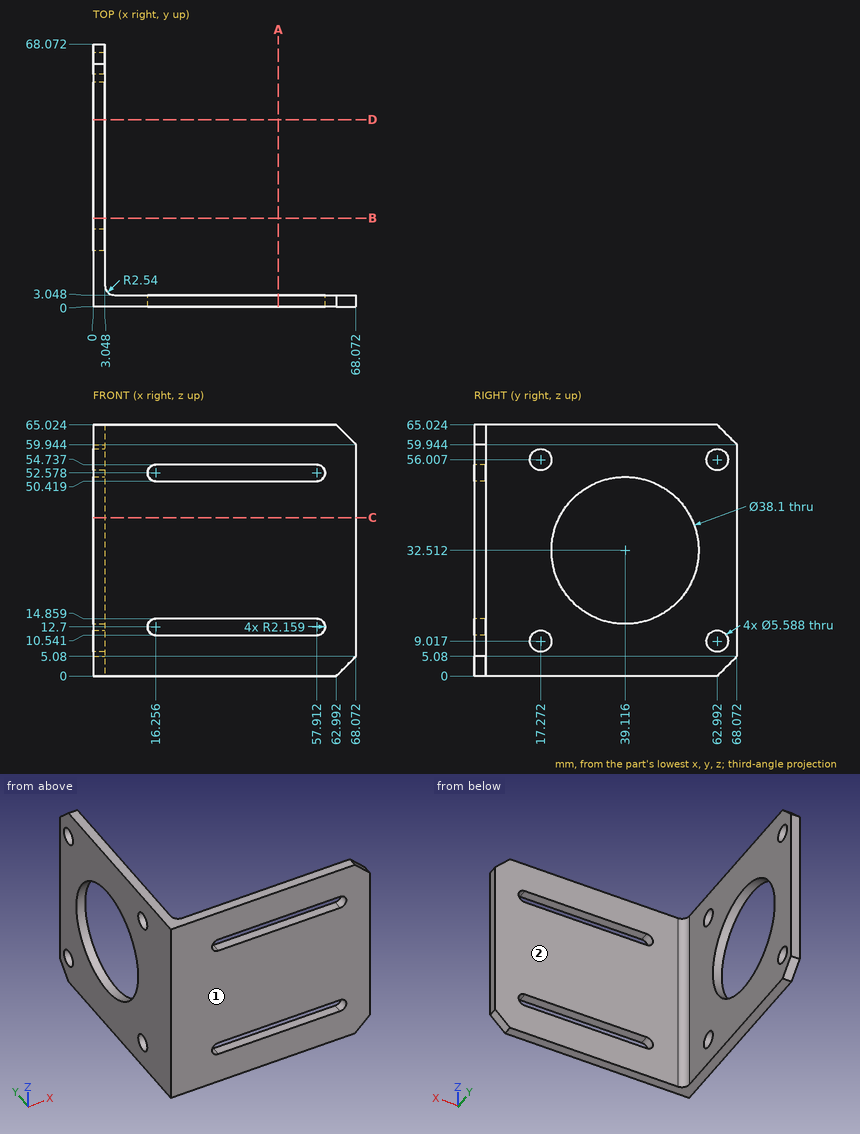
The figure shows three views and two pictorial views of one solid part (mm, origin at its lowest corner). Answer the questions. A direction names the side the tool comes from. Give positions to 0.01 mm unless a question says otherwise; leave off trailing zeros. Write each loop counter-clockwise with the first axis right and the second up, starting at its lowest first coordinate (ties: lowest second). Pieces come first, ordered by that corner, then holes. Notation, with made-up numbers: (-38.5, -12.5) - (-14.5, -12.5) arc R17 cw to (-14.5, -2.5) - close; hole circle Ø6 at (-38.75, -36). An arc over 180 degrees is marked (long way). Use CSV: the item, a comma, the result in double quotes. Start each with the question number.
Item 1: The part is cut by section A-A, the plane x = 48. Give the vertices of the cut face in (y, z).
Item 2: For the marked faces 1 and 2, determine the directions among +Z, -Z, +X, -X, +Y, -Y from which every point of the face is accessible in a straight line to the end or side of a thin tool.
Item 3: Consider line 1 (X direction, y = 61, z = 36); line 2 (X direction, y = 3.5, z = 44). Determine where each line is inside the solid, lowest interval first.
Item 4: Flat-ended cylindrical pins translate along their axes: P1, Ø1, axis at x = 25, z = 31.5, coming from the +Y side; P2, Ø9, axis at y = 62.992, z = 9.017, coming from the +X side. Find the tip coordinate at first contact, or state that the pin passes through.
Item 5: The part is cut by section B-B, the plane y = 23. Give the vertices of the cut face in (x, z), and give its area (3 significant figures).
Item 6: The part is cut by section D-D, the plane y = 48.5. Give the vertices of the cut face in (x, z), and give its area (3 significant figures).
Item 7: The part is cut by section C-C, the plane z = 41. Give the vertices of the cut face in (x, y), and give its area (3 significant figures).
Taken from the geometry:
1,outline,"(0, 0) - (3.05, 0) - (3.05, 10.54) - (0, 10.54) - close; (0, 14.86) - (3.05, 14.86) - (3.05, 50.42) - (0, 50.42) - close; (0, 54.74) - (3.05, 54.74) - (3.05, 65.02) - (0, 65.02) - close"
2,face 1,"+Z, -Z, +X, -X, -Y"
2,face 2,"+Z, -Z, +X, +Y"
3,line 1,"0 to 3.05"
3,line 2,"0 to 4.14"
4,P1,"y = 3.05"
4,P2,"x = 3.05"
5,outline,"(0, 0) - (3.05, 0) - (3.05, 22.35) - (0, 22.35) - close; (0, 42.67) - (3.05, 42.67) - (3.05, 65.02) - (0, 65.02) - close"
5,area,"136 mm2"
6,outline,"(0, 0) - (3.05, 0) - (3.05, 15.93) - (0, 15.93) - close; (0, 49.09) - (3.05, 49.09) - (3.05, 65.02) - (0, 65.02) - close"
6,area,"97.1 mm2"
7,outline,"(0, 0) - (68.07, 0) - (68.07, 3.05) - (5.59, 3.05) arc R2.54 cw to (3.05, 5.59) - (3.05, 22.06) - (0, 22.06) - close; (0, 56.17) - (3.05, 56.17) - (3.05, 68.07) - (0, 68.07) - close"
7,area,"303 mm2"
